Autodesk Inventor part; units mm, degrees
ref_plane "YZ Plane" through (0, 0, 0) normal (1, 0, 0) x (0, 1, 0)
ref_plane "XZ Plane" through (0, 0, 0) normal (0, 1, 0) x (-1, 0, 0)
ref_plane "XY Plane" through (0, 0, 0) normal (0, 0, 1) x (1, 0, 0)
sketch "スケッチ1" plane through (0, 0, 0) normal (0, 0, 1) x (1, 0, 0)
  line L0 (0, 0) -> (138, 0)
  line L1 (138, 0) -> (138, 44)
  line L2 (138, 44) -> (20, 44)
  line L3 (20, 44) -> (20, 4)
  line L4 (20, 4) -> (0, 4)
  line L5 (0, 4) -> (0, 0)
  dimension "d0" = 20
  dimension "d1" = 4
  dimension "d2" = 40
  dimension "d3" = 118
extrude "押し出し1" add sketch "スケッチ1" along normal blind 150
chamfer "面取り1" distance 5 distance2 20 1 edges at (20, 44, 75) measured on face at (98.6667, 44, 50)
chamfer "面取り2" distance 5 distance2 20 1 edges at (81.5, 44, 0) measured on face at (100.3333, 44, 50)
chamfer "面取り3" distance 5 distance2 20 1 edges at (138, 44, 77.5) measured on face at (100.3333, 44, 53.3333)
chamfer "面取り4" distance 5 distance2 20 1 edges at (79, 44, 150) measured on face at (97, 44, 101.6667)
fillet "フィレット1" radius 5 4 edges at (79, 44, 5) (25, 44, 75) (79, 44, 145) (133, 44, 75)
properties part number "おもり"
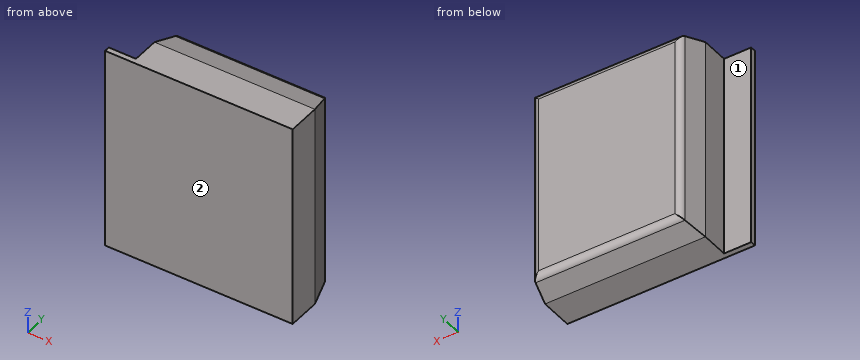
The model under review builds one solid part; all positions refer to its coordinate system, in mm. Face numbers are marked on the shaded views. A direction names the side the tool comes from. Give positions to 0.01 mm unless a question says otherwise; leave off trailing zeros. Write each loop counter-clockwise with the first axis right and the second up, starting at its lowest first coordinate (ties: lowest second). Pieces come first, ordered by that corner, then holes. Notation, with made-up numbers: M -20.75,-35 L 15.25,-35 A17 ccw 15.25,-27 Z; hole C 37,55.5 d8. An arc over 180 degrees is marked long. Write item = value, one per line. Start each with the question number.
Q1. Machinability: for the marked faces 1 and 2, which of the approach directions +Z, -Z, +X, -X, +Y, -Y give a long, thin tool a straight path to every point of the face, cutting with its end or side? Answer none if there is none.
Q2. We need section C-C (y = 30). State the section outline as (x, z) points, plus the area to 3 significant figures.
Q3. We need section A-A (z = 20.5). State the section outline as (x, y) points, plus the area to 3 significant figures.
Q4. We need section B-B (x = 122.5). State the section outline as (y, z) points.
Q5. For line 1 (X direction, y = 19.5, z = 26); line 2 (Y direction, x = 16.5, z = 113.5); line 3 (Z direction, x = 125.5, y = 24.5) (3 decimals), list the stretches that pass through material, from the lowest coordinate up.
Q6. Clearance check with flat-ended pins moving along their axes: pin 1 (4 mm diameter, centred on x = 19.5, y = 29, fed in from +Z); pin 2 (4 mm diameter, centred on y = 9, z = 128, fed in from -X); pin 3 (6 mm diameter, centred on x = 11, z = 42, fed in from +Y). State where each tip first meets the part, or that it passes through.
Q7. We need section D-D (y = 7.5). State the section outline as (x, z) points, plus the area to 3 significant figures.
Result set:
q1.face_1 = +Z, -Z, -X, +Y
q1.face_2 = +Z, -Z, +X, -X, -Y
q2.outline = M 21.5,1.5 L 136.5,1.5 L 136.5,148.5 L 21.5,148.5 Z
q2.area = 16,900 mm2
q3.outline = M 0,0 L 138,0 L 138,24 L 133.95,40.21 A5 ccw 129.1,44 L 28.9,44 A5 ccw 24.05,40.21 L 20,24 L 20,4 L 0,4 Z
q3.area = 5,170 mm2
q4.outline = M 0,0 L 24,0 L 40.21,4.05 A5 ccw 44,8.9 L 44,141.1 A5 ccw 40.21,145.95 L 24,150 L 0,150 Z
q5.line_1 = 20 to 138
q5.line_2 = 0 to 4
q5.line_3 = 0.125 to 149.875
q6.pin_1 = 149.11
q6.pin_2 = 20
q6.pin_3 = 4
q7.outline = M 20,0 L 138,0 L 138,150 L 20,150 Z
q7.area = 17,700 mm2
